Part model, mm, in its own coordinate system. Face numbers are marked on the shaded views. A direction names the side the tool comes from. Round coordinates to 2 decimals unless told otherwise and drop trailing zeros. Write each loop counter-clockwise with the first axis right and the second up, starting at its lowest first coordinate (ties: lowest second). Pieces come first, ordered by that corner, then holes. Notation, with made-up numbers: M 75,86.5 L 86,86.5 A20 cw 86,101.5 Z; hole C 0.25,13 d8. An arc over 180 degrees is marked long. Answer as a JSON object with one key per item and string values. Group by question number.
1. Band-saw the part on D-D, the plane z = -12.5. Write the cut outline in (x, y).
2. Two-plate mould, pull along X, no slides. Class the marked faces 5, 6 and 7: +X half, -X half, draft (parallel to the pull), parting line (faces both ways), or undercut.
3. Drill centre lines: line 1 (X direction, y = 12.5, z = -7.5); line 2 (Y direction, x = -8, z = 3.5); line 3 (Z direction, x = -10.5, y = -2.75). Where is each one in solid material? Low to high. Write a range as from..to.
4. Which spindle directions (+Z, -Z, +X, -X, +Y, -Y) get a long thin tool onto all of the face, cutting with end or side? Do the marked faces 1, 2, 3 and 4. Say none if no direction does.
5. Band-saw the part on C-C, the plane y = 10. Write the cut outline in (x, z).
6. Band-saw the part on B-B, the plane z = 5.5. Write the cut outline in (x, y), plus the area to 3 significant figures.
7. Drop flat-ended pins along their axis: pin 1 (4 mm diameter, centred on x = 0.5, z = 2.5, fed in from +Y); pin 2 (4 mm diameter, centred on x = 1.5, y = -0.5, fed in from +Z); pin 3 (6 mm diameter, centred on x = -9.5, z = -3, fed in from +Y); pin 4 (10 mm diameter, centred on y = 10, z = -4.5, fed in from +X). Give the stop position or say it passes through.
8. Band-saw the part on A-A, the plane x = 9.75. Write the cut outline in (y, z).
from build123d import *

# Parameters (mm, degrees)
ESBO_O1_W                  = 30
ESBO_O1_H                  = 10
RESSALTO_EXTRUS_O1_DEPTH   = 13
ESBO_O2_W                  = 30
ESBO_O2_H                  = 3.8
CORTE_EXTRUS_O1_DEPTH      = 10
FILETE1_R                  = 3
CORTE_EXTRUS_O2_DEPTH      = 23.226110771
CORTE_EXTRUS_O2_DEPTH_BACK = 23.226110771
ESBO_O3_W                  = 2.5
ESBO_O3_H                  = 4
ESBO_O4_W                  = 25
ESBO_O4_H                  = 25
RESSALTO_EXTRUS_O2_DEPTH   = 1.5
CHANFRO1_SIZE              = 5
CHANFRO1_SIZE_2            = 8.660254038
CHANFRO2_SIZE              = 7
CHANFRO2_SIZE2             = 4.041451884
ESBO_O5_R                  = 8.5
ESBO_O5_R_2                = 1
CORTE_EXTRUS_O3_DEPTH      = 3
FILETE2_R                  = 4
ESBO_O6_R                  = 1.5
RESSALTO_EXTRUS_O3_DEPTH   = 3
RESSALTO_EXTRUS_O4_START   = 0.5
ESBO_O7_R                  = 2.5
ESBO_O7_R_2                = 1.5
RESSALTO_EXTRUS_O4_DEPTH   = 0.5
CORTE_EXTRUS_O4_DEPTH      = 5


with BuildPart() as part:
    # Esboço1 → Ressalto-extrusão1 (new body)
    with BuildSketch(Plane.XY):
        Rectangle(ESBO_O1_W, ESBO_O1_H)
    extrude(amount=RESSALTO_EXTRUS_O1_DEPTH)

    # Esboço2 → Corte-extrusão1 (cut)
    with BuildSketch(Plane.XY.offset(13)):
        Rectangle(ESBO_O2_W, ESBO_O2_H)
    extrude(amount=-CORTE_EXTRUS_O1_DEPTH, mode=Mode.SUBTRACT)

    # Filete1
    filete1_edges = [part.edges().sort_by_distance(p)[0] for p in [
        (-15, 3.45, 13),
        (15, 3.45, 13),
        (-15, -3.45, 13),
        (15, -3.45, 13),
    ]]
    fillet(filete1_edges, radius=FILETE1_R)

    # Esboço3 → Corte-extrusão2 (cut, two sides: drawn at the far end of the back side and taken through both)
    with BuildSketch(Plane(origin=(0, 5, 0), x_dir=(1, 0, 0), z_dir=(0, 1, 0)).offset(-CORTE_EXTRUS_O2_DEPTH_BACK)):
        with Locations((9.906768391, -9)):
            Rectangle(ESBO_O3_W, ESBO_O3_H)
        with Locations((-9.906768391, -9)):
            Rectangle(ESBO_O3_W, ESBO_O3_H)
    extrude(amount=CORTE_EXTRUS_O2_DEPTH + CORTE_EXTRUS_O2_DEPTH_BACK, mode=Mode.SUBTRACT)

    # Esboço4 → Ressalto-extrusão2 (add, symmetric)
    with BuildSketch(Plane(origin=(13, 0, 0), x_dir=(0, 0, -1), z_dir=(1, 0, 0))):
        with Locations((12.5, 8.5)):
            Rectangle(ESBO_O4_W, ESBO_O4_H)
    extrude(amount=RESSALTO_EXTRUS_O2_DEPTH, both=True)

    # Chanfro1
    # the kernel refuses this chamfer: 8.660254038, 5 mm, written as the material it adds along each edge
    with BuildSketch(Plane(origin=(11.5, -4, 0), x_dir=(0, -0.9983227437537924, 0.05789386240267202), z_dir=(1, 0, 0))) as chanfro1_piece_1_section:
        Polygon((CHANFRO1_SIZE * 0.998322743754, CHANFRO1_SIZE * 0.0578938624027), (-CHANFRO1_SIZE_2 * 0.0578938624016, CHANFRO1_SIZE_2 * 0.998322743736), (0, 0), align=None)
    chanfro1_piece_1 = extrude(amount=3, mode=Mode.PRIVATE)
    chanfro1_piece_1 = split(chanfro1_piece_1, bisect_by=Plane(origin=(13, -5, -4.055902091), z_dir=(0, 1, 0)), keep=Keep.TOP, mode=Mode.PRIVATE)
    add(chanfro1_piece_1)

    # Chanfro2
    chanfro2_edges = [part.edges().sort_by_distance(p)[0] for p in [
        (13, 5, 0),
    ]]
    chanfro2_side = [part.faces().sort_by_distance(p)[0] for p in [
        (0, 5, 6.301932384),
    ]]
    chamfer(chanfro2_edges, length=CHANFRO2_SIZE, length2=CHANFRO2_SIZE2, reference=chanfro2_side[0])

    # Esboço5 → Corte-extrusão3 (cut)
    with BuildSketch(Plane.ZY.offset(-11.5)):
        with Locations((-12.5, 10)):
            Circle(ESBO_O5_R)
        with Locations((-20.2, 17.7)):
            Circle(ESBO_O5_R_2)
        with Locations((-4.8, 17.7)):
            Circle(ESBO_O5_R_2)
        with Locations((-4.8, 2.3)):
            Circle(ESBO_O5_R_2)
        with Locations((-20.2, 2.3)):
            Circle(ESBO_O5_R_2)
    extrude(amount=-CORTE_EXTRUS_O3_DEPTH, mode=Mode.SUBTRACT)

    # Filete2
    filete2_edges = [part.edges().sort_by_distance(p)[0] for p in [
        (13, 21, 0),
        (13, 21, -25),
        (13, -4, -25),
    ]]
    fillet(filete2_edges, radius=FILETE2_R)

    # Esboço6 → Ressalto-extrusão3 (add)
    with BuildSketch(Plane(origin=(-5, 0, 0), x_dir=(0, 0, -1), z_dir=(1, 0, 0))):
        with BuildLine():
            Line((9.606638802, 14.077800998), (-3.187293044, 5))
            Line((-3.187293044, 5), (0, 5))
            Line((0, 5), (0, -5))
            Line((0, -5), (15.393361198, 5.922199002))
            ThreePointArc((15.393361198, 5.922199002), (16.577800998, 12.893361198), (9.606638802, 14.077800998))
        make_face()
        with Locations((12.5, 10)):
            Circle(ESBO_O6_R, mode=Mode.SUBTRACT)
    ressalto_extrus_o3 = extrude(amount=-RESSALTO_EXTRUS_O3_DEPTH)

    # Esboço7 → Ressalto-extrusão4 (add)
    with BuildSketch(Plane(origin=(-5, 0, 0), x_dir=(0, 0, -1), z_dir=(1, 0, 0)).offset(RESSALTO_EXTRUS_O4_START)):
        with Locations((12.5, 10)):
            Circle(ESBO_O7_R)
        with Locations((12.5, 10)):
            Circle(ESBO_O7_R_2, mode=Mode.SUBTRACT)
    ressalto_extrus_o4 = extrude(amount=-RESSALTO_EXTRUS_O4_DEPTH)

    # Espelhar1: Ressalto-extrusão3, Ressalto-extrusão4 across plane
    add(ressalto_extrus_o3.mirror(Plane(origin=(0, 0, 0), x_dir=(0, 0, 1), z_dir=(1, 0, 0))))
    add(ressalto_extrus_o4.mirror(Plane(origin=(0, 0, 0), x_dir=(0, 0, 1), z_dir=(1, 0, 0))))

    # Esboço8 → Corte-extrusão4 (cut)
    with BuildSketch(Plane(origin=(15, 0, 0), x_dir=(0, 0, -1), z_dir=(1, 0, 0))):
        Polygon((-7.894114033, 22.521884482), (29.173309196, 22.521884482), (29.173309196, 5), (29.173309196, -5), (0, -5), (0, 5), (-7.894114033, 5), align=None)
    extrude(amount=-CORTE_EXTRUS_O4_DEPTH, mode=Mode.SUBTRACT)


solid = part.part
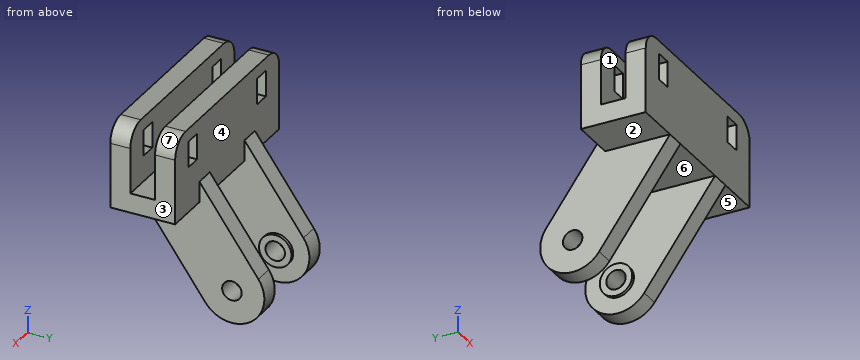
Worked answers:
{
 "1": {"outline": "M -8,3.87 L -5,3.87 L -5,7.5 L -4.5,7.5 L -4.5,8.5 L -8,8.5 Z; M -8,11.5 L -4.5,11.5 L -4.5,12.5 L -5,12.5 L -5,15 L -8,15 Z; M 4.5,7.5 L 5,7.5 L 5,3.87 L 8,3.87 L 8,8.5 L 4.5,8.5 Z; M 4.5,11.5 L 8,11.5 L 8,15 L 5,15 L 5,12.5 L 4.5,12.5 Z"},
 "2": {"face 5": "draft", "face 6": "undercut", "face 7": "+X half"},
 "3": {"line 1": "x = -8..-5, 5..8", "line 2": "y = -5..-1.9, 1.9..5", "line 3": "z = 0..7, 11..13"},
 "4": {"face 1": "+Z, +X, -X", "face 2": "-Z, -X, +Y, -Y", "face 3": "+Z, -Z, +X, +Y, -Y", "face 4": "+Z, +Y"},
 "5": {"outline": "M -8,-17.5 L -5,-17.5 L -5,-15 L -4.5,-15 L -4.5,-14 L -8,-14 Z; M -8,-11 L -4.5,-11 L -4.5,-10 L -5,-10 L -5,-3.86 L -8,-3.86 Z; M 4.5,-15 L 5,-15 L 5,-17.5 L 8,-17.5 L 8,-14 L 4.5,-14 Z; M 4.5,-11 L 8,-11 L 8,-3.86 L 5,-3.86 L 5,-10 L 4.5,-10 Z"},
 "6": {"outline": "M -15,-5 L 15,-5 L 15,-1.9 L -15,-1.9 Z; M -15,1.9 L 15,1.9 L 15,5 L -15,5 Z", "area": "186 mm^2"},
 "7": {"pin 1": "stops at y = 5", "pin 2": "stops at z = 13", "pin 3": "stops at y = 11.23", "pin 4": "stops at x = 8"},
 "8": {"outline": "M -5,0 L 5,0 L 5,7 L 1.9,7 L 1.9,3 L -1.9,3 L -1.9,7 L -5,7 Z; M -5,11 L -1.9,11 L -1.9,13 L -5,13 Z; M 1.9,11 L 5,11 L 5,13 L 1.9,13 Z"}
}
